Autodesk Fusion 360 part; units mm, degrees
sketch "Sketch1" plane through (0, 0, 0) normal (0, 0, 1) x (1, 0, 0)
  line L0 (-35, 57) -> (35, 57)
  line L1 (35, 57) -> (35, -57)
  line L2 (35, -57) -> (-35, -57)
  line L3 (-35, -57) -> (-35, 57)
  line L4 (-50, 0) -> (50, 0)
  circle A0 centre (0.0006, 30.16) radius 3.5
  circle A1 centre (0.0006, -30.16) radius 3.5
  line L5 (0, 65) -> (0, -65)
  line L6 (5.155, 0) -> (5.155, 11.965)
  line L7 (5.155, 11.965) -> (0, 11.965)
  line L8 (-5.155, 11.965) -> (0, 11.965)
  line L9 (-5.155, 0) -> (-5.155, 11.965)
  line L10 (-5.155, 0) -> (-5.155, -11.965)
  line L11 (5.155, -11.965) -> (0, -11.965)
  line L12 (5.155, 0) -> (5.155, -11.965)
  line L13 (-5.155, -11.965) -> (0, -11.965)
  circle A2 centre (0.0006, 30.16) radius 2.25
  circle A3 centre (0.0006, -30.16) radius 2.25
  circle A4 centre (0.0006, 30.16) radius 5
  circle A5 centre (0.0006, -30.16) radius 5
  circle A6 centre (21, 45) radius 2.5
  circle A7 centre (-21, 45) radius 2.5
  circle A8 centre (21, -45) radius 2.5
  circle A9 centre (-21, -45) radius 2.5
  circle A10 centre (16, 0) radius 2.5
  circle A11 centre (-16, 0) radius 2.5
  line L14 (31, 53) -> (-31, 53)
  line L15 (-31, 53) -> (-31, -53)
  line L16 (-31, -53) -> (31, -53)
  line L17 (31, -53) -> (31, 53)
  dimension "d1" = 60.32
  dimension "d3" = 10.31
  dimension "d4" = 23.93
  dimension "d5" = 4.5
  dimension "d6" = 10
  dimension "d7" = 5
  dimension "d8" = 114
  dimension "d9" = 5
  dimension "d24" = 7
extrude "Extrude1" add sketch "Sketch1" along normal blind 5.5 contours L0 L3 L4 L5 L14 L15 | L0 L1 L4 L5 L14 L17 | L2 L3 L4 L5 L15 L16 | L1 L2 L4 L5 L16 L17 makes body 1
extrude "Extrude2" add sketch "Sketch1" along normal blind 3 separate body contours L4 A11 | L4 A11 | L4 A10 | L4 A10 | A6 | A7 | A8 | A9 makes body 2 at (23.4969, -45.1246, 2) makes body 3 at (-13.5124, -0.2489, 1) makes body 4 at (-18.5031, 44.8754, 2) makes body 5 at (-18.5031, -45.1246, 2) makes body 6 at (18.4876, -0.2489, 1) makes body 7 at (23.4969, 44.8754, 2)
extrude "Extrude3" add sketch "Sketch1" along normal blind 2 contours L4 L5 L6 L7 A4 A10 L14 L17 | L4 L5 L8 L9 A4 A11 L14 L15 | L4 L5 L10 L13 A5 A11 L15 L16 | L4 L5 L11 L12 A5 A10 L16 L17 bodies 1 2 3 4 5 6 7
chamfer "Chamfer1" distance 2.5 distance2 3.5 4 edges at (-31, 0, 5.5) (0, 53, 5.5) (31, 0, 5.5) (0, -53, 5.5) measured on face at (33.6667, -17.6667, 5.5) measured on face at (33.6667, -17.6667, 5.5) measured on face at (33.6667, -17.6667, 5.5) measured on face at (33.6667, -17.6667, 5.5) on bodies 1
chamfer "Chamfer2" distance 2 distance2 3.5 4 edges at (35, 0, 0) (0, -57, 0) (-35, 0, 0) (0, 57, 0) measured on face at (-25.0517, 3.9883, 0) measured on face at (-25.0517, 3.9883, 0) measured on face at (-25.0517, 3.9883, 0) measured on face at (-25.0517, 3.9883, 0) on bodies 1
extrude "Extrude4" add sketch "Sketch1" along normal blind 4 contours A0 L5 A4 | A0 L5 A4 | A0 L5 A2 | A0 L5 A2 | A1 L5 A5 | A1 L5 A5 | A1 L5 A3 | A1 L5 A3 bodies 1
chamfer "Chamfer3" distance 2.5 distance2 1.25 2 edges at (-2.0971, -29.3464, 0) (-2.0971, 30.9736, 0) measured on face at (2.2394, -29.936, 2.6667) measured on face at (2.2394, 30.384, 1.3333) on bodies 1
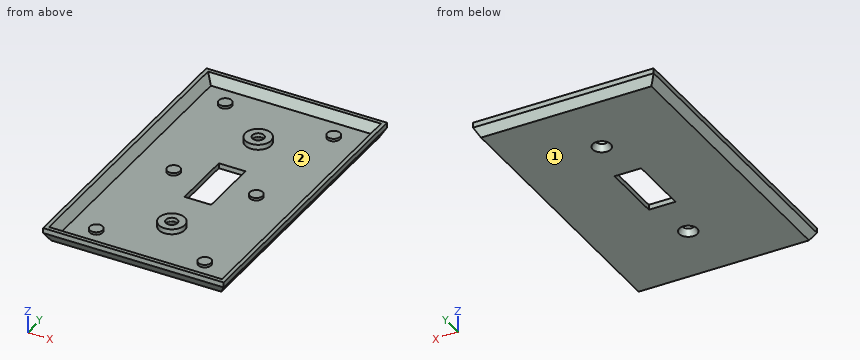
Design review of the part built by this model. Coordinates are the model's own, in mm. Face numbers are marked on the shaded views. Give positions to 0.01 mm unless a question says otherwise; leave off trailing zeros. Return JSON: item names as keys, results as strings. Group by question number.
(1) Mouldability with a two-part tool opening along Y and no side actions: class the marked faces 1 and 2 as +Y half, -Y half, draft (parallel to the pull), parting line (faces both ways), or undercut.
(2) To check wall thickness, follow probe 1 along X at (y, z) = (30.16, 3.75); probe 2 along X at (y, z) = (36, 3.95); probe 3 along X at (y, z) = (30.16, 3.55). State the ranges of each line that lie inside material, in increasing order.
(3) Insertion check: pin 1 (3 mm diameter, centred on x = -1.5, y = -28, fed in from +Z); pin 2 (1.5 mm diameter, centred on x = 20.5, y = -44.5, fed in from +Z); pin 3 (3 mm diameter, centred on x = -26.5, y = -14.5, fed in from +Z); pin 4 (3.5 mm diameter, centred on x = 0, y = -30.16, fed in from +Z). Each pin has a flat end and moves straight along its axis. Give the tip position at first contact, or say it passes through.
Reported:
{
 "1": {"face 1": "draft", "face 2": "undercut"},
 "2": {"probe 1": "x = -35 to -32.25, -5 to -2.25, 2.25 to 5, 32.25 to 35", "probe 2": "x = -35 to -32.39, 32.39 to 35", "probe 3": "x = -35 to -32.11, -5 to -2.25, 2.25 to 5, 32.11 to 35"},
 "3": {"pin 1": "stops at z = 4", "pin 2": "stops at z = 3", "pin 3": "stops at z = 2", "pin 4": "passes through"}
}
